Build history of the part. All positions in model axes, mm. A direction names the side the tool comes from. Coordinates: 2 decimals unless noted, no trailing zeros. Order: outer loops, then holes, each group sorted by start corner. A loop starts at its lowest first (then second) coordinate and runs counter-clockwise, first axis right, second up. Notation, with made-up numbers: (74.5, 57.5) - (119.5, 57.5) arc R20 ccw to (119.5, 67.5) - close; hole circle Ø1 at (82, -27.5). An arc over 180 degrees is marked (long way). One line per item, written item: value.
Autodesk Inventor part; units mm, degrees
ref_plane "YZ Plane" through (0, 0, 0) normal (1, 0, 0) x (0, 1, 0)
ref_plane "XZ Plane" through (0, 0, 0) normal (0, 1, 0) x (-1, 0, 0)
ref_plane "XY Plane" through (0, 0, 0) normal (0, 0, 1) x (1, 0, 0)
sketch "Sketch1" plane through (0, 0, 0) normal (0, 0, 1) x (1, 0, 0)
  circle A0 centre (0, 0) radius 15.875
  circle A1 centre (0, 0) radius 3.175
  dimension "d0" = 31.75
  dimension "d1" = 6.35
extrude "Extrusion1" add sketch "Sketch1" along normal blind 34.925
sketch "Sketch2" plane through (0, 0, 34.925) normal (0, 0, 1) x (1, 0, 0)
  circle A0 centre (0, 0) radius 15.875
  circle A1 centre (0, 0) radius 6.35
  circle A2 centre (0, 0) radius 12.7
  dimension "d4" = 6.35
  dimension "d5" = 12.7
extrude "Extrusion2" cut sketch "Sketch2" against normal blind 11.1125 contours A2
sketch "Sketch3" plane through (0, 0, 0) normal (0, 0, -1) x (-1, 0, 0)
  circle A0 centre (0, 0) radius 15.875
  circle A1 centre (0, 0) radius 6.35
  circle A2 centre (0, 0) radius 12.7
  dimension "d8" = 12.7
  dimension "d9" = 6.35
extrude "Extrusion3" cut sketch "Sketch3" against normal blind 11.1125 contours A2
fillet "Fillet1" radius 0.7937 4 edges at (6.35, 0, 0) (-15.875, 0, 0) (-6.35, 0, 34.925) (-15.875, 0, 34.925)
properties part number "Conveyor_Roller_MainOuter" material "PVC-Piping"
1. Band-saw the part on C-C, the plane z = 25.5. Give the cut face in (x, y) (3 decimals), and give its area (3 significant figures).
Values found:
outline: circle Ø31.75 at (0, 0); circle Ø12.7 at (0, 0); hole circle Ø25.4 at (0, 0); hole circle Ø6.35 at (0, 0)
area: 380 mm2
2. Probe line 1 along Y through (x, z) = (0, 29) (3 decimals); line 2 along Y through (x, z) = (-1.5, 33); line 3 along Y through (x, z) = (0, 19) (3 decimals). List the from-to ranges inside material, lowest first.
Values found:
line 1: y = -15.875 to -12.7, -6.35 to -3.175, 3.175 to 6.35, 12.7 to 15.875
line 2: y = -15.8 to -12.61, -6.17 to -2.8, 2.8 to 6.17, 12.61 to 15.8
line 3: y = -15.875 to -3.175, 3.175 to 15.875
3. Band-saw the part on D-D, the plane z = 21. Give the cut face in (x, y) (3 decimals).
Values found:
outline: circle Ø31.75 at (0, 0); hole circle Ø6.35 at (0, 0)
4. Flat gauge pins, fed straight in: P1, Ø1, axis at x = 10.5, z = 16.5, coming from the -Y side; P2, Ø1.5, axis at x = 8.5, z = 29.5, coming from the +Y side; P3, Ø8, axis at x = -7.5, z = 12, coming from the -Y side; P4, Ø5, axis at x = 0, y = 0, coming from the -Z side (1 decimal). Where does each tip first touch, or does it go through?
Values found:
P1: stops at y = -12.33
P2: stops at y = 13.85
P3: stops at y = -15.48
P4: passes through
5. 3-axis set-ups, long thin cutter, end or side, ignore diameter. For faces 4 (the face through (-2.75, -12.4, 29.45)), 5 (the face through (-7, -11, 0)), 6 (the face through (2.75, -12.4, 5.48)): which of +Z, -Z, +X, -X, +Y, -Y reach the whole face in a straight line?
Values found:
face 4: +Z
face 5: -Z, +X, -X, +Y, -Y
face 6: -Z
6. Two-plate mould, pull along X, no slides. Class faces 1 (the face through (2.4, -2.4, 0)), 2 (the face through (-3.441, 15.497, 17.229)), 3 (the face through (-1.38, -6.2, 29.04)): pulls with the +X half, pulls with the -X half, needs draft (parallel to the pull), parting line crosses it, or undercut.
Values found:
face 1: needs draft
face 2: parting line crosses it
face 3: undercut
